```python
from build123d import *

# Parameters (mm, degrees)
SKETCH_R     = 21
PAD_DEPTH    = 2
SKETCH001_R  = 7
PAD001_DEPTH = 7
SKETCH002_R  = 3.5
HOLE_DEPTH   = 7.001
POCKET_DEPTH = 4.5
CHAMFER_SIZE = 1


with BuildPart() as part:
    # Sketch → Pad (new body)
    with BuildSketch(Plane.XY):
        Circle(SKETCH_R)
    extrude(amount=PAD_DEPTH)

    # Sketch001 → Pad001 (join)
    with BuildSketch(Plane.XY):
        Circle(SKETCH001_R)
    extrude(amount=PAD001_DEPTH)

    # Sketch002 → Hole (cut, through all)
    with BuildSketch(Plane.XY):
        Circle(SKETCH002_R)
    extrude(amount=HOLE_DEPTH, mode=Mode.SUBTRACT)

    # Sketch003 → Pocket (cut)
    with BuildSketch(Plane.XY):
        Polygon((2.670245, -4.625), (5.34049, 0), (2.670245, 4.625), (-2.670245, 4.625), (-5.34049, 0), (-2.670245, -4.625), align=None)
    extrude(amount=POCKET_DEPTH, mode=Mode.SUBTRACT)

    # Chamfer
    chamfer_edges = [part.edges().sort_by_distance(p)[0] for p in [
        (-4.005367, -2.3125, 4.5),
        (0, -4.625, 4.5),
        (4.005367, -2.3125, 4.5),
        (4.005367, 2.3125, 4.5),
        (0, 4.625, 4.5),
        (-4.005367, 2.3125, 4.5),
    ]]
    chamfer(chamfer_edges, length=CHAMFER_SIZE)


solid = part.part
```
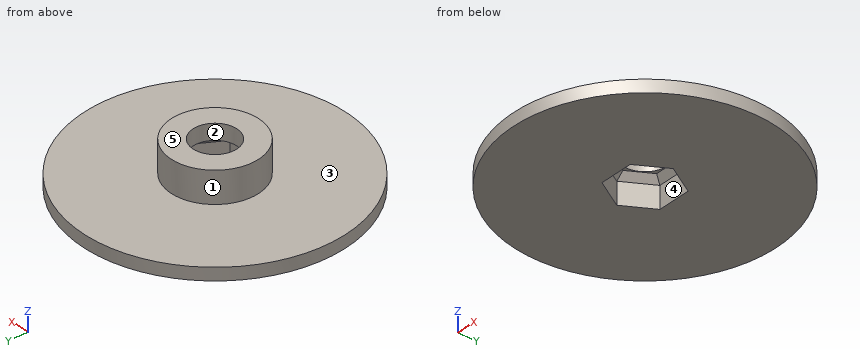
For this review, take the finished solid that the model builds, in its own axes (mm). Face numbers are marked on the shaded views. A direction names the side the tool comes from. Coordinates: 2 decimals unless noted, no trailing zeros. Write each loop counter-clockwise with the first axis right and the second up, starting at its lowest first coordinate (ties: lowest second). Pieces come first, ordered by that corner, then holes.
(1) For pin 1 Ø1 at (x, z) = (6.5, 5) entering from +Y; pin 2 Ø1 at (x, z) = (0.5, 5.5) entering from -Y; pin 3 Ø12 at (x, y) = (1.5, 14.5) entering from +Z, all flat-tipped, find the tip position at first contact; note any pin that passes through.
(2) Add section C-C on y = -2.5. Give the boundary of the cut face in (x, z).
(3) Add section D-D on x = -6. Give the boundary of the cut face in (y, z), then the cut area to 3 significant figures.
(4) Wall thickness on probe 1 along Y at (x, z) = (0, 5.15); probe 2 along Z at (x, y) = (13, -12.5): over which ranges is each line inside the solid? List them lowest first.
(5) Add section A-A on x = 0. Give the boundary of the cut face in (y, z) (3 decimals), then the cut area to 3 significant figures.
(6) Add section B-B on z = 1.25. Give the boundary of the cut face in (x, y) (3 decimals), then the cut area to 3 significant figures.
(7) Tool access review of the marked faces 4 and 5: name each direction out of +Z, -Z, +X, -X, +Y, -Y from which nothing blocks a thin tool from reaching the whole face with its end or side.
(8) The part is to be moulded in two halves that separate along Y. For the marked faces 1, 2 and 3, say which applies: +Y half, -Y half, draft (parallel to the pull), parting line (faces both ways), or undercut.
Answer sheet:
1. pin 1: stops at y = 3.61
1. pin 2: stops at y = -7
1. pin 3: stops at z = 2
2. outline: (-20.85, 0) - (-3.9, 0) - (-3.9, 3.5) - (-2.74, 4.5) - (-2.45, 4.5) - (-2.45, 7) - (-6.54, 7) - (-6.54, 2) - (-20.85, 2) - close; (2.45, 4.5) - (2.74, 4.5) - (3.9, 3.5) - (3.9, 0) - (20.85, 0) - (20.85, 2) - (6.54, 2) - (6.54, 7) - (2.45, 7) - close
3. outline: (-20.12, 0) - (20.12, 0) - (20.12, 2) - (3.61, 2) - (3.61, 7) - (-3.61, 7) - (-3.61, 2) - (-20.12, 2) - close
3. area: 117 mm2
4. probe 1: y = -7 to -3.5, 3.5 to 7
4. probe 2: z = 0 to 2
5. outline: (-21, 0) - (-4.625, 0) - (-4.625, 3.5) - (-3.625, 4.5) - (-3.5, 4.5) - (-3.5, 7) - (-7, 7) - (-7, 2) - (-21, 2) - close; (3.5, 4.5) - (3.625, 4.5) - (4.625, 3.5) - (4.625, 0) - (21, 0) - (21, 2) - (7, 2) - (7, 7) - (3.5, 7) - close
5. area: 95.9 mm2
6. outline: circle Ø42 at (0, 0); hole (-5.34, 0) - (-2.67, -4.625) - (2.67, -4.625) - (5.34, 0) - (2.67, 4.625) - (-2.67, 4.625) - close
6. area: 1,310 mm2
7. face 4: -Z
7. face 5: +Z, +X, -X, +Y, -Y
8. face 1: parting line
8. face 2: undercut
8. face 3: draft
